CAD build for the part. Positions are in the model's coordinates, mm. Face numbers are marked on the shaded views. A direction names the side the tool comes from. Round coordinates to 2 decimals unless told otherwise and drop trailing zeros. Loops run counter-clockwise (first coordinate to the right, second up) from the corner with the lowest first, then second, coordinate; pieces in that order, holes last. Notation, with made-up numbers: (-5.5, 12.25) - (40.5, 12.25) arc R21 cw to (40.5, 30.25) - close; hole circle Ø1 at (-2, 41.5). An arc over 180 degrees is marked (long way). Use one line per item in the form item = value.
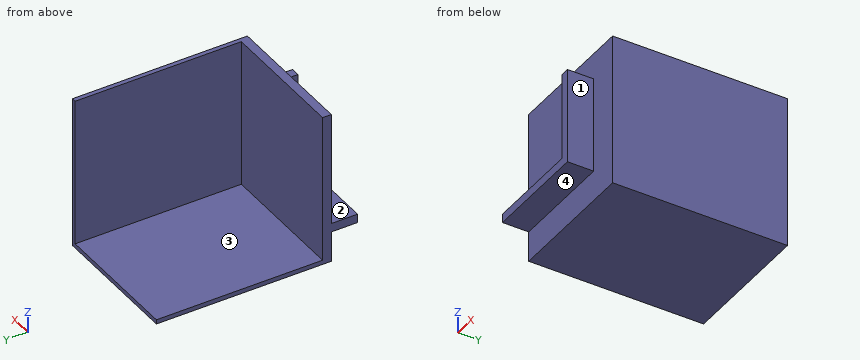
from build123d import *

# Parameters (mm, degrees)
SKETCH1_W               = 150
SKETCH1_H               = 10
BOSS_EXTRUDE1_DEPTH     = 200
BOSS_EXTRUDE2_DEPTH     = 205
SKETCH3_W               = 5
SKETCH3_H               = 300
BOSS_EXTRUDE3_DEPTH     = 150
BOSS_EXTRUDE4_DEPTH     = 30
CUT_EXTRUDE3_DEPTH      = 151
CUT_EXTRUDE3_DEPTH_BACK = 6


with BuildPart() as part:
    # Sketch1 → Boss-Extrude1 (new body)
    with BuildSketch(Plane.XY):
        with Locations((-9.782608696, -38.260869565)):
            Rectangle(SKETCH1_W, SKETCH1_H)
    extrude(amount=-BOSS_EXTRUDE1_DEPTH)

    # Sketch2 → Boss-Extrude2 (add)
    with BuildSketch(Plane.XY):
        Polygon((65.217391304, -43.260869565), (70.217391304, -43.260869565), (70.217391304, 256.739130435), (65.217391304, 256.739130435), (65.217391304, -33.260869565), align=None)
    extrude(amount=-BOSS_EXTRUDE2_DEPTH)

    # Sketch3 → Boss-Extrude3 (add)
    with BuildSketch(Plane.ZY.offset(84.782608696)):
        with Locations((-202.5, 106.739130435)):
            Rectangle(SKETCH3_W, SKETCH3_H)
    extrude(amount=-BOSS_EXTRUDE3_DEPTH)

    # Sketch4 → Boss-Extrude4 (add)
    with BuildSketch(Plane.XZ.offset(43.260869565)):
        Polygon((25.217391304, -160), (-84.782608696, -160), (-84.782608696, -170), (35.217391304, -170), (35.217391304, -60), (25.217391304, -60), align=None)
    extrude(amount=BOSS_EXTRUDE4_DEPTH)

    # Sketch5 → Cut-Extrude3 (cut, two sides)
    with BuildSketch(Plane.ZY.offset(-65.217391304)) as cut_extrude3_sk:
        Polygon((-205, 256.739130435), (-205, 156.739130435), (-30, 156.739130435), (-30, -73.260869565), (0, -73.260869565), (0, 256.739130435), align=None)
    extrude(amount=CUT_EXTRUDE3_DEPTH, mode=Mode.SUBTRACT)
    extrude(cut_extrude3_sk.sketch, amount=-CUT_EXTRUDE3_DEPTH_BACK, mode=Mode.SUBTRACT)


solid = part.part
1) Slice it at B-B (x = -40). Write the cut outline in (y, z).
Report:
outline = (-73.26, -170) - (-43.26, -170) - (-43.26, -205) - (156.74, -205) - (156.74, -200) - (-33.26, -200) - (-33.26, -30) - (-43.26, -30) - (-43.26, -160) - (-73.26, -160) - close
2) Slice it at D-D (z = -176.5). Write the cut outline in (x, y).
Report:
outline = (-84.78, -43.26) - (70.22, -43.26) - (70.22, 156.74) - (65.22, 156.74) - (65.22, -33.26) - (-84.78, -33.26) - close
3) Slice it at C-C (y = 33). Write the cut outline in (x, z).
Report:
outline = (-84.78, -205) - (70.22, -205) - (70.22, -30) - (65.22, -30) - (65.22, -200) - (-84.78, -200) - close
4) Slice it at A-A (z = -93). Write the cut outline in (x, y).
Report:
outline = (-84.78, -43.26) - (25.22, -43.26) - (25.22, -73.26) - (35.22, -73.26) - (35.22, -43.26) - (70.22, -43.26) - (70.22, 156.74) - (65.22, 156.74) - (65.22, -33.26) - (-84.78, -33.26) - close
5) Drill centre lines: probe 1 along Y at (x, z) = (39, -115.5); probe 2 along Y at (x, z) = (-45, -165.5); probe 3 along Z at (x, y) = (-59, -3). Where is each one in solid material? Low to high.
Report:
probe_1 = -43.26 to -33.26
probe_2 = -73.26 to -33.26
probe_3 = -205 to -200
6) Flat gauge pins, fed straight in: pin 1 (1 mm diameter, centred on x = 28.5, z = -186.5, fed in from +Y); pin 2 (24 mm diameter, centred on y = -65.5, z = -128, fed in from +X); pin 3 (1.5 mm diameter, centred on x = 51.5, z = -134, fed in from -Y). Where does each tip first touch, or does it go through?
Report:
pin_1 = -33.26
pin_2 = 35.22
pin_3 = -43.26
7) Tool access for the marked faces 1, 2, 3 and 4: list every direction of +Z, -Z, +X, -X, +Y, -Y with a clear straight run to the whole face (end or side of a thin tool).
Report:
face_1 = +Z, -Z, +X, -Y
face_2 = +Z, -X, -Y
face_3 = +Z, -X, +Y
face_4 = -Z, +X, -X, -Y
